```python
from build123d import *

# Parameters (mm, degrees)
CYLINDER271_R          = 2.5
CYLINDER271_DEPTH      = 19.2
CYLINDER272_R          = 6.1
CYLINDER272_DEPTH      = 7.2
CYLINDER273_R          = 7.95
CYLINDER273_DEPTH      = 1.3
CYLINDER270_R          = 7.95
CYLINDER270_DEPTH      = 7.5
CUT197_ROLL_ANGLE      = -90
CUT197_PLACEMENT_ANGLE = 90


with BuildPart() as cylinder271:
    # Cylinder271 → Cylinder271 (new body)
    with BuildSketch(Plane.XY.offset(-2)):
        Circle(CYLINDER271_R)
    extrude(amount=CYLINDER271_DEPTH)


with BuildPart() as cylinder272:
    # Cylinder272 → Cylinder272 (new body)
    with BuildSketch(Plane.XY.offset(7)):
        Circle(CYLINDER272_R)
    extrude(amount=CYLINDER272_DEPTH)


with BuildPart() as cylinder273:
    # Cylinder273 → Cylinder273 (new body)
    with BuildSketch(Plane.XY.offset(14)):
        Circle(CYLINDER273_R)
    extrude(amount=CYLINDER273_DEPTH)


with BuildPart() as cut197:
    # Cylinder270 → Cylinder270 (new body)
    with BuildSketch(Plane.XY):
        Circle(CYLINDER270_R)
    extrude(amount=CYLINDER270_DEPTH)

    # Fusion105: union Cylinder272, Cylinder273
    add(cylinder272.part)
    add(cylinder273.part)

    # Cut197: cut Cylinder271
    add(cylinder271.part, mode=Mode.SUBTRACT)


with BuildPart() as cut197_1:
    # Cut197 roll: moved
    add(cut197.part.rotate(Axis((0, 0, 0), (1, 0, 0)), CUT197_ROLL_ANGLE))


with BuildPart() as cut197_2:
    # Cut197 placement: moved
    add(cut197_1.part.moved(Location((88.85, 182.14, 155.15))).rotate(Axis((88.85, 182.14, 155.15), (0, 0, 1)), CUT197_PLACEMENT_ANGLE))


solid = cut197_2.part
```
Source: CAD feature listing. Evaluate the final solid. Frame: model axes, mm. A direction names the side the tool comes from. Give positions to 0.01 mm unless a question says otherwise; leave off trailing zeros. Loops run counter-clockwise (first coordinate to the right, second up) from the corner with the lowest first, then second, coordinate; pieces in that order, holes last. Notation, with made-up numbers: (10.25, 19.25) - (59.25, 19.25) arc R12 ccw to (59.25, 41.25) - close; hole circle Ø11 at (14, 22). An arc over 180 degrees is marked (long way). Use CSV: the item, a comma, the result in double quotes. Start each with the question number.
1. Pin query (flat end, axial travel): pin 1 (1.5 mm diameter, centred on x = 78, y = 178, fed in from -Z); pin 2 (3 mm diameter, centred on y = 182.14, z = 155.15, fed in from +X); pin 3 (1.5 mm diameter, centred on x = 84, y = 180, fed in from -Z); pin 4 (1.5 mm diameter, centred on x = 80, y = 186, fed in from -Z). Return the tip coordinate at first contact, or that it passes through.
2. Section C-C (x = 76.5). Output: boundary loops of the cut face in (y, z), then the cut area to 3 significant figures.
3. Reachability of faces 5 (the cylindrical face through (74.209, 181.105, 147.268)), 6 (the flat face through (81.35, 184.5, 161)) from +Z, -Z, +X, -X, +Y, -Y: full face, straight path, thin tool, end or side. Return the list, or none.
4. Section A-A (z = 155.15). Output: boundary loops of the cut face in (x, y), then the cut area to 3 significant figures.
5. Section B-B (y = 182.14). Output: boundary loops of the cut face in (x, z), then the cut area to 3 significant figures.
6. Draft query along X for faces 1 (the flat face through (74.85, 184.5, 161)), 2 (the flat face through (88.85, 180, 157)), 3 (the cylindrical face through (78.15, 177.3, 158.86)), 4 (the cylindrical face through (85.153, 181.105, 147.268)). Return one class per face: +X half, -X half, draft (parallel to the pull), parting line (faces both ways), or undercut.
7. Section D-D (z = 150.5). Output: boundary loops of the cut face in (x, y), then the cut area to 3 significant figures.
8. Ray query, L1, parallel to Z at x = 80.25, y = 182.14; L2, parallel to X at y = 176, z = 158; L3, parallel to Y at x = 83, z = 155.15. Return the intervals inside material, ascending.
Response:
1,pin 1,"z = 150.08"
1,pin 2,"through"
1,pin 3,"z = 147.32"
1,pin 4,"z = 149.9"
2,outline,"circle Ø12.2 at (182.14, 155.15); hole circle Ø5 at (182.14, 155.15)"
2,area,"97.3 mm²"
3,face 5,"+X, -X"
3,face 6,"none"
4,outline,"(73.55, 174.19) - (74.85, 174.19) - (74.85, 176.04) - (81.35, 176.04) - (81.35, 174.19) - (88.85, 174.19) - (88.85, 179.64) - (73.55, 179.64) - close; (73.55, 184.64) - (88.85, 184.64) - (88.85, 190.09) - (81.35, 190.09) - (81.35, 188.24) - (74.85, 188.24) - (74.85, 190.09) - (73.55, 190.09) - close"
4,area,"143 mm²"
5,outline,"(73.55, 147.2) - (74.85, 147.2) - (74.85, 149.05) - (81.35, 149.05) - (81.35, 147.2) - (88.85, 147.2) - (88.85, 152.65) - (73.55, 152.65) - close; (73.55, 157.65) - (88.85, 157.65) - (88.85, 163.1) - (81.35, 163.1) - (81.35, 161.25) - (74.85, 161.25) - (74.85, 163.1) - (73.55, 163.1) - close"
5,area,"143 mm²"
6,face 1,"undercut"
6,face 2,"+X half"
6,face 3,"undercut"
6,face 4,"draft"
7,outline,"(73.55, 175.69) - (74.85, 175.69) - (74.85, 178.19) - (81.35, 178.19) - (81.35, 175.69) - (88.85, 175.69) - (88.85, 188.59) - (81.35, 188.59) - (81.35, 186.09) - (74.85, 186.09) - (74.85, 188.59) - (73.55, 188.59) - close"
7,area,"165 mm²"
8,L1,"149.05 to 152.65, 157.65 to 161.25"
8,L2,"73.55 to 74.85, 81.35 to 88.85"
8,L3,"174.19 to 179.64, 184.64 to 190.09"
